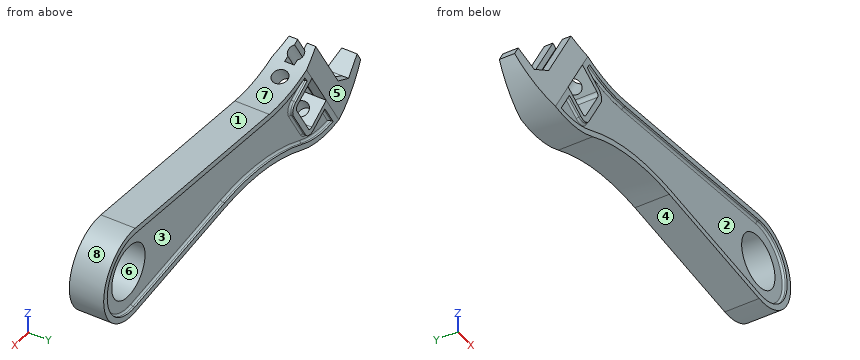
```python
from build123d import *

# Parameters (mm, degrees)
SKETCH1_R               = 7
BOSS_EXTRUDE1_DEPTH     = 4.5
CUT_EXTRUDE1_DEPTH      = 93.949210636
CUT_EXTRUDE1_DEPTH_BACK = 4
SKETCH2_R               = 2
CUT_EXTRUDE2_DEPTH      = 94.860420286
CUT_EXTRUDE3_DEPTH      = 94.860420286
CUT_EXTRUDE3_DEPTH_BACK = 94.860420286
FILLET1_R               = 1
CUT_EXTRUDE4_START      = -1
CUT_EXTRUDE4_DEPTH      = 103.671038166
FILLET2_R               = 0.5
FILLET2_OF_MIRROR1_R    = 0.5


with BuildPart() as part:
    # Sketch1 → Boss-Extrude1 (new, symmetric)
    with BuildSketch(Plane(origin=(0, 0, 0), x_dir=(1, 0, 0), z_dir=(0, 1, 0))):
        with BuildLine():
            Line((-1.254341559, 11.934262744), (-38.985522111, 7.968555867))
            ThreePointArc((-38.985522111, 7.968555867), (-55.482588048, 8.517606008), (-71.205780018, 13.541138114))
            ThreePointArc((-71.205780018, 13.541138114), (-86.438642867, 15.605996242), (-100, 8.367671688))
            Line((-100, 8.367671688), (-98.5, 5.769595477))
            Line((-98.5, 5.769595477), (-93.303847577, 8.769595477))
            Line((-93.303847577, 8.769595477), (-88.107695155, 5.769595477))
            Line((-88.107695155, 5.769595477), (-78.705771366, -10.515014214))
            ThreePointArc((-78.705771366, -10.515014214), (-68.482680545, -6.590737321), (-57.547275152, -6.017637008))
            Line((-57.547275152, -6.017637008), (-1.254341559, -11.934262744))
            ThreePointArc((-1.254341559, -11.934262744), (12, 0), (-1.254341559, 11.934262744))
        make_face()
        with Locations(Location((0, 0, 0), (0, 0, 270))):
            Circle(SKETCH1_R, mode=Mode.SUBTRACT)
        Polygon((-81.509618943, 6.341392247), (-75.509618943, -4.050912599), (-68.581415713, -0.050912599), (-74.581415713, 10.341392247), align=None, mode=Mode.SUBTRACT)
    extrude(amount=BOSS_EXTRUDE1_DEPTH, both=True)

    # Sketch2 → Cut-Extrude1 (cut, two sides: drawn at the far end of the back side and taken through both)
    with BuildSketch(Plane(origin=(-23.123308126, 0, -40.050744514), x_dir=(0.86602540378444, 0, -0.49999999999999784), z_dir=(0.49999999999999784, 0, 0.86602540378444)).offset(-CUT_EXTRUDE1_DEPTH_BACK)):
        with Locations(Location((-63.418704534, 0, 0), (0, 0, 180))):
            Circle(SKETCH2_R)
    extrude(amount=CUT_EXTRUDE1_DEPTH + CUT_EXTRUDE1_DEPTH_BACK, mode=Mode.SUBTRACT)

    # Sketch3 → Cut-Extrude2 (cut, through all)
    with BuildSketch(Plane(origin=(-27.123308126, 0, -46.978947744), x_dir=(0.8660254037844406, 0, -0.4999999999999967), z_dir=(0.4999999999999967, 0, 0.8660254037844406))):
        with BuildLine():
            Line((-82.418704534, -1.25), (-71.979954034, -1.25))
            ThreePointArc((-71.979954034, -1.25), (-70.418704534, -2), (-68.857455035, -1.25))
            Line((-68.857455035, -1.25), (-67.418704534, -1.25))
            Line((-67.418704534, -1.25), (-67.418704534, 1.25))
            Line((-67.418704534, 1.25), (-68.857455035, 1.25))
            ThreePointArc((-68.857455035, 1.25), (-70.418704534, 2), (-71.979954034, 1.25))
            Line((-71.979954034, 1.25), (-82.418704534, 1.25))
            Line((-82.418704534, 1.25), (-82.418704534, -1.25))
        make_face()
    extrude(amount=CUT_EXTRUDE2_DEPTH, mode=Mode.SUBTRACT)

    # Sketch4 → Cut-Extrude3 (cut, two sides: drawn at the far end of the back side and taken through both)
    with BuildSketch(Plane(origin=(-27.123308126, 0, -46.978947744), x_dir=(0.8660254037844406, 0, -0.4999999999999967), z_dir=(0.4999999999999967, 0, 0.8660254037844406)).offset(-CUT_EXTRUDE3_DEPTH_BACK)):
        Polygon((-82.418704534, 4.5), (-82.418704534, 2), (-67.418704534, 4.5), align=None)
        Polygon((-82.418704534, -4.5), (-82.418704534, -2), (-67.418704534, -4.5), align=None)
    extrude(amount=CUT_EXTRUDE3_DEPTH + CUT_EXTRUDE3_DEPTH_BACK, mode=Mode.SUBTRACT)

    # Fillet1
    fillet1_edges = [part.edges().sort_by_distance(p)[0] for p in [
        (-74.581415713, 0, -10.341392247),
        (-68.581415713, 0, 0.050912599),
    ]]
    fillet(fillet1_edges, radius=FILLET1_R)

    # Sketch5 → Cut-Extrude4 (cut)
    with BuildSketch(Plane(origin=(0, 4.5, 0), x_dir=(1, 0, 0), z_dir=(0, 1, 0)).offset(CUT_EXTRUDE4_START)):
        with BuildLine():
            Line((-84.417038698, 14.377190981), (-80.960580838, 8.390430352))
            Line((-80.960580838, 8.390430352), (-76.197441117, 11.140430352))
            ThreePointArc((-76.197441117, 11.140430352), (-74.300393504, 11.390181409), (-72.782377607, 10.225366843))
            Line((-72.782377607, 10.225366843), (-67.782377607, 1.565112805))
            ThreePointArc((-67.782377607, 1.565112805), (-67.532626551, -0.331934808), (-68.697441117, -1.849950704))
            Line((-68.697441117, -1.849950704), (-73.460580838, -4.599950704))
            Line((-73.460580838, -4.599950704), (-72.571151937, -6.14048675))
            ThreePointArc((-72.571151937, -6.14048675), (-65.066176866, -4.530624461), (-57.390482457, -4.525854165))
            Line((-57.390482457, -4.525854165), (-1.097548864, -10.442479901))
            ThreePointArc((-1.097548864, -10.442479901), (10.5, 0), (-1.097548864, 10.442479901))
            Line((-1.097548864, 10.442479901), (-38.828729416, 6.476773024))
            ThreePointArc((-38.828729416, 6.476773024), (-55.738222001, 7.039549419), (-71.854493771, 12.188669828))
            ThreePointArc((-71.854493771, 12.188669828), (-77.984484997, 14.151314674), (-84.417038698, 14.377190981))
        make_face()
    cut_extrude4 = extrude(amount=CUT_EXTRUDE4_DEPTH, mode=Mode.SUBTRACT)

    # Fillet2
    fillet2_edges = [part.edges().sort_by_distance(p)[0] for p in [
        (-78.579010977, 3.5, -9.765430352),
        (-74.300393504, 3.5, -11.390181409),
        (-71.079010977, 3.5, 3.224950704),
        (-67.532626551, 3.5, 0.331934808),
        (-65.066176866, 3.5, 4.530624461),
        (-29.24401566, 3.5, 7.484167033),
        (10.5, 3.5, 0),
        (-19.96313914, 3.5, -8.459626463),
        (-55.738222001, 3.5, -7.039549419),
        (-73.015866387, 3.5, 5.370218727),
        (-70.282377607, 3.5, -5.895239824),
        (-82.688809768, 3.5, -11.383810667),
        (-77.984484997, 3.5, -14.151314674),
    ]]
    fillet(fillet2_edges, radius=FILLET2_R)

    # Mirror1: Cut-Extrude4 across plane
    add(cut_extrude4.mirror(Plane.ZX), mode=Mode.SUBTRACT)

    # Fillet2 of Mirror1
    fillet2_of_mirror1_edges = [part.edges().sort_by_distance(p)[0] for p in [
        (-78.579010977, -3.5, -9.765430352),
        (-74.300393504, -3.5, -11.390181409),
        (-71.079010977, -3.5, 3.224950704),
        (-67.532626551, -3.5, 0.331934808),
        (-65.066176866, -3.5, 4.530624461),
        (-29.24401566, -3.5, 7.484167033),
        (10.5, -3.5, 0),
        (-19.96313914, -3.5, -8.459626463),
        (-55.738222001, -3.5, -7.039549419),
        (-73.015866387, -3.5, 5.370218727),
        (-70.282377607, -3.5, -5.895239824),
        (-82.688809768, -3.5, -11.383810667),
        (-77.984484997, -3.5, -14.151314674),
    ]]
    fillet(fillet2_of_mirror1_edges, radius=FILLET2_OF_MIRROR1_R)


solid = part.part
```
Work out the finished part from the listing and answer in its coordinate system (mm). Face numbers are marked on the shaded views. A direction names the side the tool comes from. Coordinates: 2 decimals unless noted, no trailing zeros. Answer as a JSON object with one key per item and string values.
Q1. Which of the six approach directions +Z, -Z, +X, -X, +Y, -Y give full straight-line access (tool end or side, diameter ignored) to the marked faces 1, 2, 3, 4 and 5?
Results list:
{"face 1": "+Z, +Y, -Y", "face 2": "-Y", "face 3": "+Y", "face 4": "-Z, +Y, -Y", "face 5": "+Z, -X, +Y"}
Q2. Consider L1, parallel to Z at x = 0, y = 4.4; L2, parallel to Y at x = -37, z = 6.25; L3, parallel to X at y = 1.5, z = 0.5. Determine where each line is inside the solid, lowest interval first. Write a range as from..to.
Results list:
{"L1": "z = -12..-10.5, 10.5..12", "L2": "y = -3.51..3.51", "L3": "x = -84.49..-82.55, -79.5..-77.56, -69.37..-6.98, 6.98..11.99"}
Q3. Given pin 1 Ø2 at (y, z) = (-2.5, 6) entering from +X; pin 2 Ø7 at (x, z) = (-14, -5) entering from -Y; pin 3 Ø12 at (x, z) = (-50.5, -0.5) entering from +Y; pin 4 Ø4 at (x, z) = (-83, 1.5) entering from -Y, each flat-ended and moving along its own axis, determine where each tip first touches the part or whether it passes through.
Results list:
{"pin 1": "stops at x = 10.91", "pin 2": "stops at y = -3.5", "pin 3": "stops at y = 4.5", "pin 4": "stops at y = -3.96"}
Q4. For a pull along Z with two mould halves and no side action, classify the marked faces 6, 7 and 8 as pulls with the +Z half, pulls with the -Z half, needs draft (parallel to the pull), parting line crosses it, or undercut.
Results list:
{"face 6": "undercut", "face 7": "pulls with the +Z half", "face 8": "parting line crosses it"}
